Geometry check sheet. Reference: drawing and pictorial views, mm from the part's lowest x, y, z. A direction names the side the tool comes from. Round coordinates to 2 decimals unless told otherwise and drop trailing zeros. Order: outer loops, then holes, each group sorted by start corner. A loop starts at its lowest first (then second) coordinate and runs counter-clockwise, first axis right, second up.
(1) Cross-section at B-B on z = 82.5. Enter the section's corners in (x, y).
(2) Gauge pin test, flat ends, axial feed: P1, Ø7.5, axis at y = 8, z = 9.5, coming from the +X side; P2, Ø12, axis at x = 99, z = 42.5, coming from the -Y side; P3, Ø8, axis at x = 84.5, y = 20, coming from the +Z side; P4, Ø12, axis at x = 98, y = 9.5, coming from the +Z side. Record the tip position at first contact, or that the pin passes through.
(3) Cross-section at A-A on y = 4. Enter the section's corners in (x, z) (1 decimal).
(4) Cross-section at C-C on z = 19. Enter the section's corners in (x, y).
(5) Thickness scan on L1, parallel to X at y = 13.75, z = 30; L2, parallel to X at y = 8, z = 13.5 (1 decimal); L3, parallel to X at y = 17, z = 81.5 (1 decimal). Record the ranges inside material, lowest first.
(6) Cross-section at D-D on x = 74. Enter the section's corners in (y, z) (1 decimal).
(7) Set-up check for the marked faces 1, 2, 3 and 4: record each of +Z, -Z, +X, -X, +Y, -Y from which the full face is reachable in a straight line by a thin tool's end or side.
(8) Draft check along X on the marked faces 5, 6 and 7. Enter one of: pulls with the +X half, pulls with the -X half, needs draft (parallel to the pull), parting line crosses it, or undercut.
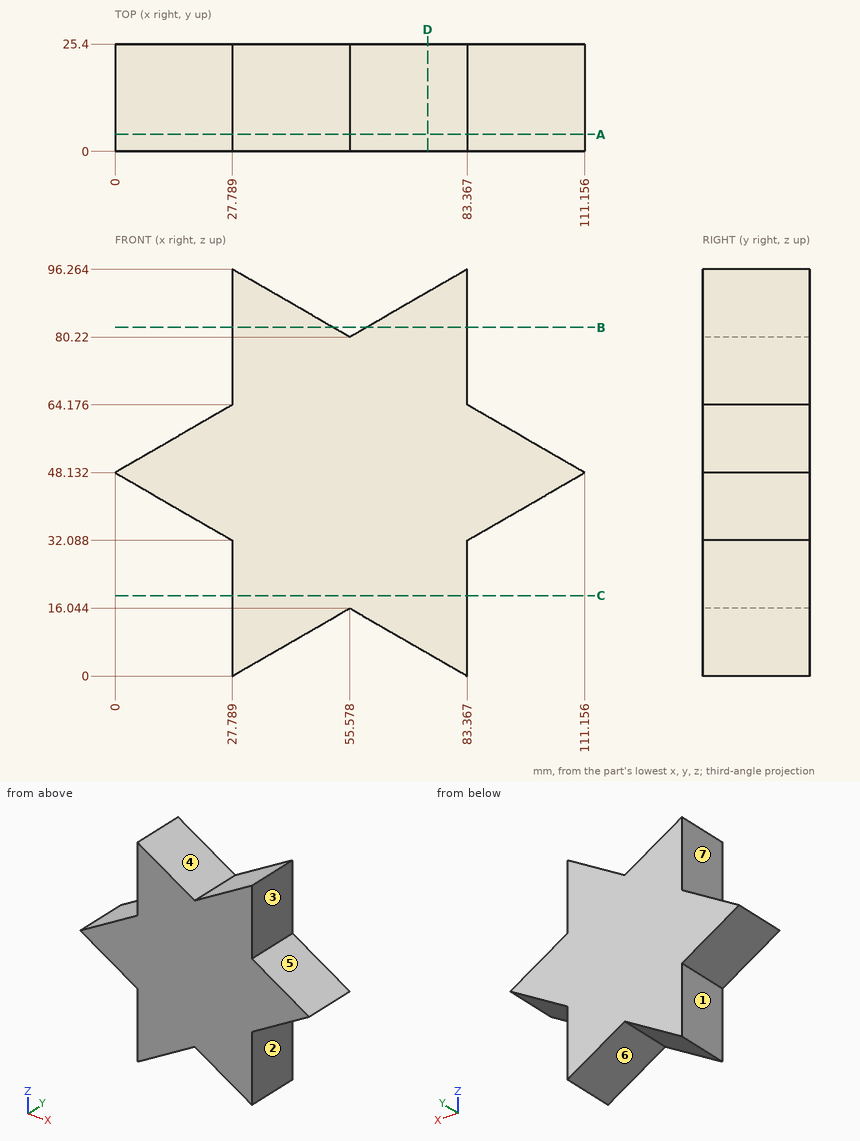
Found:
1. outline: (27.79, 0) - (51.63, 0) - (51.63, 25.4) - (27.79, 25.4) - close; (59.53, 0) - (83.37, 0) - (83.37, 25.4) - (59.53, 25.4) - close
2. P1: stops at x = 83.37
2. P2: stops at y = 0
2. P3: stops at z = 96.26
2. P4: stops at z = 59.19
3. outline: (0, 48.1) - (27.8, 32.1) - (27.8, 0) - (55.6, 16) - (83.4, 0) - (83.4, 32.1) - (111.2, 48.1) - (83.4, 64.2) - (83.4, 96.3) - (55.6, 80.2) - (27.8, 96.3) - (27.8, 64.2) - close
4. outline: (27.79, 0) - (83.37, 0) - (83.37, 25.4) - (27.79, 25.4) - close
5. L1: x = 27.79 to 83.37
5. L2: x = 27.8 to 51.2, 60 to 83.4
5. L3: x = 27.8 to 53.4, 57.8 to 83.4
6. outline: (0, 5.4) - (25.4, 5.4) - (25.4, 90.9) - (0, 90.9) - close
7. face 1: -Z, -X, +Y, -Y
7. face 2: -Z, +X, +Y, -Y
7. face 3: +Z, +X, +Y, -Y
7. face 4: +Z, +Y, -Y
8. face 5: pulls with the +X half
8. face 6: undercut
8. face 7: pulls with the -X half
